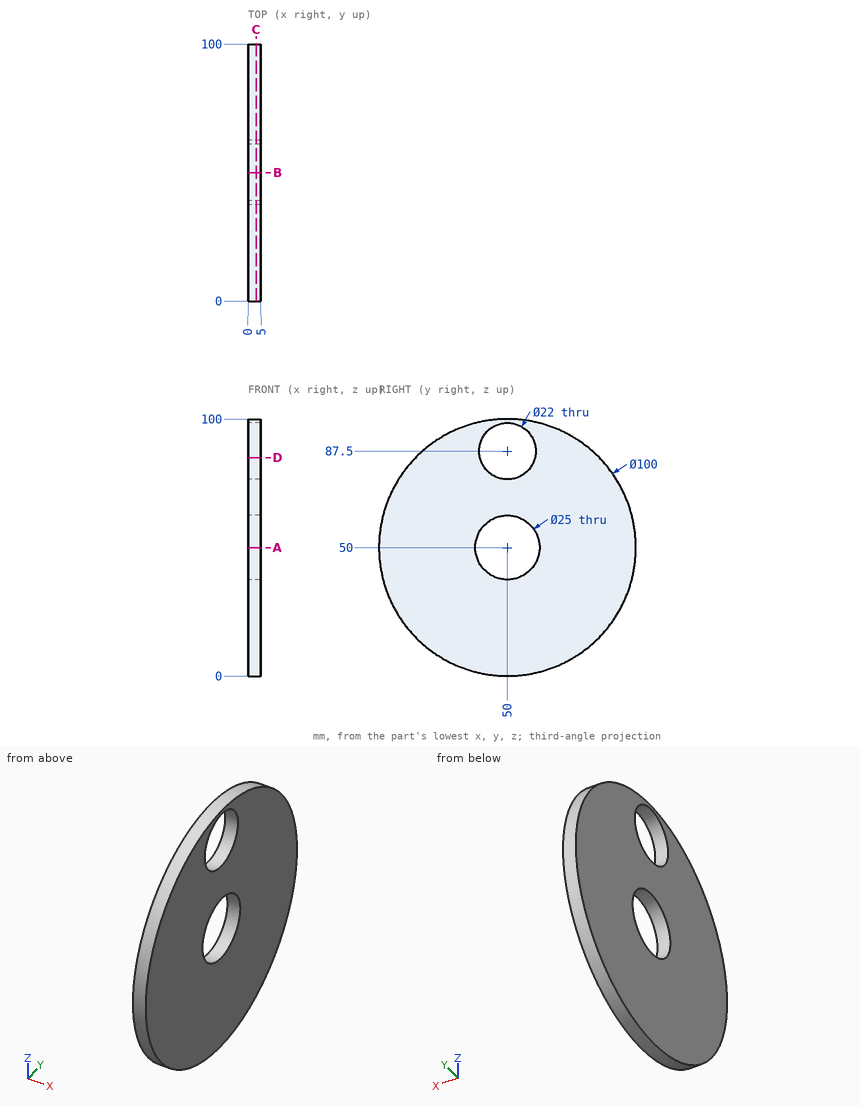
Check sheet for the drawn part. Datum: minimum x, y, z corner. Units: mm. Coordinates: 2 decimals unless noted, no trailing zeros. Order: outer loops, then holes, each group sorted by start corner. A loop starts at its lowest first (then second) coordinate and runs counter-clockwise, first axis right, second up. Notation, with made-up numbers: M 46.25,-4 L 66.25,-4 A16 ccw 66.25,12 Z; hole C 13,78 d2. An arc over 180 degrees is marked long. One line per question, with ' | ' between items. Start each with the question number.
Item 1: Gauge pin test, flat ends, axial feed: P1, Ø1, axis at x = 1.5, z = 70, coming from the -Y side; P2, Ø2, axis at x = 1.5, z = 74, coming from the -Y side. Record the tip position at first contact, or that the pin passes through.
Item 2: Sectioned sample at C-C on x = 3.15. Record the cut outline in (y, z).
Item 3: Sectioned sample at D-D on z = 85. Record the cut outline in (x, y), and give its area (3 significant figures).
Item 4: Sectioned sample at B-B on y = 50. Record the cut outline in (x, z), and give its area (3 significant figures).
Item 5: Sectioned sample at A-A on z = 50. Record the cut outline in (x, y), and give its area (3 significant figures).
Item 6: Material ranges on line 1 (Z direction, x = 3.25, y = 50); line 2 (Z direction, x = 1.85, y = 46.5); line 3 (Y direction, x = 2.8, z = 86.5), recorded low to high.
Answer below:
1) P1: stops at y = 3.96 | P2: stops at y = 5.6
2) outline: C 50,50 d100; hole C 50,50 d25; hole C 50,87.5 d22
3) outline: M 0,14.29 L 5,14.29 L 5,39.29 L 0,39.29 Z; M 0,60.71 L 5,60.71 L 5,85.71 L 0,85.71 Z | area: 250 mm^2
4) outline: M 0,0 L 5,0 L 5,37.5 L 0,37.5 Z; M 0,62.5 L 5,62.5 L 5,76.5 L 0,76.5 Z; M 0,98.5 L 5,98.5 L 5,100 L 0,100 Z | area: 265 mm^2
5) outline: M 0,0 L 5,0 L 5,37.5 L 0,37.5 Z; M 0,62.5 L 5,62.5 L 5,100 L 0,100 Z | area: 375 mm^2
6) line 1: z = 0 to 37.5, 62.5 to 76.5, 98.5 to 100 | line 2: z = 0.12 to 38, 62 to 77.07, 97.93 to 99.88 | line 3: y = 15.83 to 39.05, 60.95 to 84.17
